Model file for the job. Use its own axes, mm. A direction names the side the tool comes from. Round coordinates to 2 decimals unless told otherwise and drop trailing zeros. Loops run counter-clockwise (first coordinate to the right, second up) from the corner with the lowest first, then second, coordinate; pieces in that order, holes last.
from build123d import *

# Parameters (mm, degrees)
SKETCH1_R           = 2.325
BOSS_EXTRUDE1_DEPTH = 16.05
SKETCH1_3_W         = 4.825
SKETCH1_3_H         = 6.325
SKETCH1_3_R         = 2.325
BOSS_EXTRUDE2_DEPTH = 2.35
SKETCH1_4_R         = 2.325
BOSS_EXTRUDE3_DEPTH = 6.6
SKETCH1_5_R         = 2.325
BOSS_EXTRUDE4_DEPTH = 10.8
SKETCH1_6_R         = 2.325
BOSS_EXTRUDE5_DEPTH = 13.8


with BuildPart() as part:
    # Sketch1 → Boss-Extrude1 (new body)
    # profile 1 of 8: a face of its own
    with BuildSketch(Plane(origin=(0, 0, 0), x_dir=(1, 0, 0), z_dir=(0, 1, 0))):
        with BuildLine():
            Line((-11.4, 0), (-1.25, 0))
            ThreePointArc((-1.25, 0), (-0.929373406, 1.988246715), (0, 3.774917218))
            Line((0, 3.774917218), (0, 6.325))
            Line((0, 6.325), (-11.4, 6.325))
            Line((-11.4, 6.325), (-11.4, 0))
        make_face()
    # profile 2 of 8: a face of its own
    with BuildSketch(Plane(origin=(0, 0, 0), x_dir=(1, 0, 0), z_dir=(0, 1, 0))):
        with BuildLine():
            ThreePointArc((5.075000013, -6.325), (0.602549614, -4.472450396), (-1.25, 0))
            Line((-1.25, 0), (-11.4, 0))
            Line((-11.4, 0), (-11.4, -6.325))
            Line((-11.4, -6.325), (5.075000013, -6.325))
        make_face()
    # profile 3 of 8: a face of its own
    with BuildSketch(Plane(origin=(0, 0, 0), x_dir=(1, 0, 0), z_dir=(0, 1, 0))):
        with BuildLine():
            Line((0, 3.774917218), (0, 0))
            Line((0, 0), (-1.25, 0))
            ThreePointArc((-1.25, 0), (0.602549614, -4.472450396), (5.075000013, -6.325))
            ThreePointArc((5.075000013, -6.325), (9.547450396, -4.472450386), (11.4, 0))
            ThreePointArc((11.4, 0), (9.547450389, 4.472450393), (5.074999993, 6.325))
            ThreePointArc((5.074999993, 6.325), (2.23516958, 5.651635886), (0, 3.774917218))
        make_face()
        with Locations((5.075, 0)):
            Circle(SKETCH1_R, mode=Mode.SUBTRACT)
    # profile 4 of 8: a face of its own
    with BuildSketch(Plane(origin=(0, 0, 0), x_dir=(1, 0, 0), z_dir=(0, 1, 0))):
        with BuildLine():
            Line((-1.25, 0), (0, 0))
            Line((0, 0), (0, 3.774917218))
            ThreePointArc((0, 3.774917218), (-0.929373406, 1.988246715), (-1.25, 0))
        make_face()
    # profile 5 of 8: a face of its own
    with BuildSketch(Plane(origin=(0, 0, 0), x_dir=(1, 0, 0), z_dir=(0, 1, 0))):
        with BuildLine():
            Line((0, 6.325), (0, 3.774917218))
            ThreePointArc((0, 3.774917218), (2.23516958, 5.651635886), (5.074999993, 6.325))
            Line((5.074999993, 6.325), (0, 6.325))
        make_face()
    # profile 6 of 8: a face of its own
    with BuildSketch(Plane(origin=(0, 0, 0), x_dir=(1, 0, 0), z_dir=(0, 1, 0))):
        with BuildLine():
            Line((11.4, 6.325), (5.074999993, 6.325))
            ThreePointArc((5.074999993, 6.325), (9.547450389, 4.472450393), (11.4, 0))
            Line((11.4, 0), (11.4, 6.325))
        make_face()
    # profile 7 of 8: a face of its own
    with BuildSketch(Plane(origin=(0, 0, 0), x_dir=(1, 0, 0), z_dir=(0, 1, 0))):
        with BuildLine():
            ThreePointArc((11.4, 0), (9.547450396, -4.472450386), (5.075000013, -6.325))
            Line((5.075000013, -6.325), (11.4, -6.325))
            Line((11.4, -6.325), (11.4, 0))
        make_face()
    # profile 8 of 8: a face of its own
    with BuildSketch(Plane(origin=(0, 0, 0), x_dir=(1, 0, 0), z_dir=(0, 1, 0))):
        with Locations((5.075, 0)):
            Circle(SKETCH1_R)
    extrude(amount=-BOSS_EXTRUDE1_DEPTH)

    # Sketch1_3 → Boss-Extrude2 (add)
    # profile 1 of 11: a face of its own
    with BuildSketch(Plane(origin=(0, 0, 0), x_dir=(1, 0, 0), z_dir=(0, 1, 0))):
        with Locations((-13.8125, -3.1625)):
            Rectangle(SKETCH1_3_W, SKETCH1_3_H)
    # profile 2 of 11: a face of its own
    with BuildSketch(Plane(origin=(0, 0, 0), x_dir=(1, 0, 0), z_dir=(0, 1, 0))):
        with BuildLine():
            ThreePointArc((5.075000013, -6.325), (0.602549614, -4.472450396), (-1.25, 0))
            Line((-1.25, 0), (-11.4, 0))
            Line((-11.4, 0), (-11.4, -6.325))
            Line((-11.4, -6.325), (5.075000013, -6.325))
        make_face()
    # profile 3 of 11: a face of its own
    with BuildSketch(Plane(origin=(0, 0, 0), x_dir=(1, 0, 0), z_dir=(0, 1, 0))):
        with BuildLine():
            Line((-11.4, 0), (-1.25, 0))
            ThreePointArc((-1.25, 0), (-0.929373406, 1.988246715), (0, 3.774917218))
            Line((0, 3.774917218), (0, 6.325))
            Line((0, 6.325), (-11.4, 6.325))
            Line((-11.4, 6.325), (-11.4, 0))
        make_face()
    # profile 4 of 11: a face of its own
    with BuildSketch(Plane(origin=(0, 0, 0), x_dir=(1, 0, 0), z_dir=(0, 1, 0))):
        with Locations((-13.8125, 3.1625)):
            Rectangle(SKETCH1_3_W, SKETCH1_3_H)
    # profile 5 of 11: a face of its own
    with BuildSketch(Plane(origin=(0, 0, 0), x_dir=(1, 0, 0), z_dir=(0, 1, 0))):
        with BuildLine():
            Line((0, 3.774917218), (0, 0))
            Line((0, 0), (-1.25, 0))
            ThreePointArc((-1.25, 0), (0.602549614, -4.472450396), (5.075000013, -6.325))
            ThreePointArc((5.075000013, -6.325), (9.547450396, -4.472450386), (11.4, 0))
            ThreePointArc((11.4, 0), (9.547450389, 4.472450393), (5.074999993, 6.325))
            ThreePointArc((5.074999993, 6.325), (2.23516958, 5.651635886), (0, 3.774917218))
        make_face()
        with Locations((5.075, 0)):
            Circle(SKETCH1_3_R, mode=Mode.SUBTRACT)
    # profile 6 of 11: a face of its own
    with BuildSketch(Plane(origin=(0, 0, 0), x_dir=(1, 0, 0), z_dir=(0, 1, 0))):
        with Locations((5.075, 0)):
            Circle(SKETCH1_3_R)
    # profile 7 of 11: a face of its own
    with BuildSketch(Plane(origin=(0, 0, 0), x_dir=(1, 0, 0), z_dir=(0, 1, 0))):
        with BuildLine():
            Line((-1.25, 0), (0, 0))
            Line((0, 0), (0, 3.774917218))
            ThreePointArc((0, 3.774917218), (-0.929373406, 1.988246715), (-1.25, 0))
        make_face()
    # profile 8 of 11: a face of its own
    with BuildSketch(Plane(origin=(0, 0, 0), x_dir=(1, 0, 0), z_dir=(0, 1, 0))):
        with BuildLine():
            Line((0, 6.325), (0, 3.774917218))
            ThreePointArc((0, 3.774917218), (2.23516958, 5.651635886), (5.074999993, 6.325))
            Line((5.074999993, 6.325), (0, 6.325))
        make_face()
    # profile 9 of 11: a face of its own
    with BuildSketch(Plane(origin=(0, 0, 0), x_dir=(1, 0, 0), z_dir=(0, 1, 0))):
        with BuildLine():
            Line((11.4, 6.325), (5.074999993, 6.325))
            ThreePointArc((5.074999993, 6.325), (9.547450389, 4.472450393), (11.4, 0))
            Line((11.4, 0), (11.4, 6.325))
        make_face()
    # profile 10 of 11: a face of its own
    with BuildSketch(Plane(origin=(0, 0, 0), x_dir=(1, 0, 0), z_dir=(0, 1, 0))):
        with BuildLine():
            ThreePointArc((11.4, 0), (9.547450396, -4.472450386), (5.075000013, -6.325))
            Line((5.075000013, -6.325), (11.4, -6.325))
            Line((11.4, -6.325), (11.4, 0))
        make_face()
    # profile 11 of 11: a face of its own
    with BuildSketch(Plane(origin=(0, 0, 0), x_dir=(1, 0, 0), z_dir=(0, 1, 0))):
        Polygon((11.4, 0), (11.4, -6.325), (16.225, -6.325), (16.225, 6.325), (11.4, 6.325), align=None)
    extrude(amount=BOSS_EXTRUDE2_DEPTH)

    # Sketch1_4 → Boss-Extrude3 (add)
    # profile 1 of 8: a face of its own
    with BuildSketch(Plane(origin=(0, 0, 0), x_dir=(1, 0, 0), z_dir=(0, 1, 0))):
        with BuildLine():
            Line((-11.4, 0), (-1.25, 0))
            ThreePointArc((-1.25, 0), (-0.929373406, 1.988246715), (0, 3.774917218))
            Line((0, 3.774917218), (0, 6.325))
            Line((0, 6.325), (-11.4, 6.325))
            Line((-11.4, 6.325), (-11.4, 0))
        make_face()
    # profile 2 of 8: a face of its own
    with BuildSketch(Plane(origin=(0, 0, 0), x_dir=(1, 0, 0), z_dir=(0, 1, 0))):
        with BuildLine():
            ThreePointArc((5.075000013, -6.325), (0.602549614, -4.472450396), (-1.25, 0))
            Line((-1.25, 0), (-11.4, 0))
            Line((-11.4, 0), (-11.4, -6.325))
            Line((-11.4, -6.325), (5.075000013, -6.325))
        make_face()
    # profile 3 of 8: a face of its own
    with BuildSketch(Plane(origin=(0, 0, 0), x_dir=(1, 0, 0), z_dir=(0, 1, 0))):
        with BuildLine():
            Line((0, 3.774917218), (0, 0))
            Line((0, 0), (-1.25, 0))
            ThreePointArc((-1.25, 0), (0.602549614, -4.472450396), (5.075000013, -6.325))
            ThreePointArc((5.075000013, -6.325), (9.547450396, -4.472450386), (11.4, 0))
            ThreePointArc((11.4, 0), (9.547450389, 4.472450393), (5.074999993, 6.325))
            ThreePointArc((5.074999993, 6.325), (2.23516958, 5.651635886), (0, 3.774917218))
        make_face()
        with Locations((5.075, 0)):
            Circle(SKETCH1_4_R, mode=Mode.SUBTRACT)
    # profile 4 of 8: a face of its own
    with BuildSketch(Plane(origin=(0, 0, 0), x_dir=(1, 0, 0), z_dir=(0, 1, 0))):
        with BuildLine():
            Line((0, 6.325), (0, 3.774917218))
            ThreePointArc((0, 3.774917218), (2.23516958, 5.651635886), (5.074999993, 6.325))
            Line((5.074999993, 6.325), (0, 6.325))
        make_face()
    # profile 5 of 8: a face of its own
    with BuildSketch(Plane(origin=(0, 0, 0), x_dir=(1, 0, 0), z_dir=(0, 1, 0))):
        with BuildLine():
            Line((11.4, 6.325), (5.074999993, 6.325))
            ThreePointArc((5.074999993, 6.325), (9.547450389, 4.472450393), (11.4, 0))
            Line((11.4, 0), (11.4, 6.325))
        make_face()
    # profile 6 of 8: a face of its own
    with BuildSketch(Plane(origin=(0, 0, 0), x_dir=(1, 0, 0), z_dir=(0, 1, 0))):
        with BuildLine():
            ThreePointArc((11.4, 0), (9.547450396, -4.472450386), (5.075000013, -6.325))
            Line((5.075000013, -6.325), (11.4, -6.325))
            Line((11.4, -6.325), (11.4, 0))
        make_face()
    # profile 7 of 8: a face of its own
    with BuildSketch(Plane(origin=(0, 0, 0), x_dir=(1, 0, 0), z_dir=(0, 1, 0))):
        with BuildLine():
            Line((-1.25, 0), (0, 0))
            Line((0, 0), (0, 3.774917218))
            ThreePointArc((0, 3.774917218), (-0.929373406, 1.988246715), (-1.25, 0))
        make_face()
    # profile 8 of 8: a face of its own
    with BuildSketch(Plane(origin=(0, 0, 0), x_dir=(1, 0, 0), z_dir=(0, 1, 0))):
        with Locations((5.075, 0)):
            Circle(SKETCH1_4_R)
    extrude(amount=BOSS_EXTRUDE3_DEPTH)

    # Sketch1_5 → Boss-Extrude4 (add)
    # profile 1 of 3: a face of its own
    with BuildSketch(Plane(origin=(0, 0, 0), x_dir=(1, 0, 0), z_dir=(0, 1, 0))):
        with BuildLine():
            Line((0, 3.774917218), (0, 0))
            Line((0, 0), (-1.25, 0))
            ThreePointArc((-1.25, 0), (0.602549614, -4.472450396), (5.075000013, -6.325))
            ThreePointArc((5.075000013, -6.325), (9.547450396, -4.472450386), (11.4, 0))
            ThreePointArc((11.4, 0), (9.547450389, 4.472450393), (5.074999993, 6.325))
            ThreePointArc((5.074999993, 6.325), (2.23516958, 5.651635886), (0, 3.774917218))
        make_face()
        with Locations((5.075, 0)):
            Circle(SKETCH1_5_R, mode=Mode.SUBTRACT)
    # profile 2 of 3: a face of its own
    with BuildSketch(Plane(origin=(0, 0, 0), x_dir=(1, 0, 0), z_dir=(0, 1, 0))):
        with Locations((5.075, 0)):
            Circle(SKETCH1_5_R)
    # profile 3 of 3: a face of its own
    with BuildSketch(Plane(origin=(0, 0, 0), x_dir=(1, 0, 0), z_dir=(0, 1, 0))):
        with BuildLine():
            Line((-1.25, 0), (0, 0))
            Line((0, 0), (0, 3.774917218))
            ThreePointArc((0, 3.774917218), (-0.929373406, 1.988246715), (-1.25, 0))
        make_face()
    extrude(amount=BOSS_EXTRUDE4_DEPTH)

    # Sketch1_6 → Boss-Extrude5 (add)
    with BuildSketch(Plane(origin=(0, 0, 0), x_dir=(1, 0, 0), z_dir=(0, 1, 0))):
        with Locations(Location((5.075, 0, 0), (0, 0, 90))):
            Circle(SKETCH1_6_R)
    extrude(amount=BOSS_EXTRUDE5_DEPTH)


solid = part.part
Q1. Slice it at A-A on z = -1. Give the cut face in (x, y) (3 decimals), plus the area to 3 significant figures.
Q2. Slice it at B-B on x = 6.5. Give the cut face in (y, z) (3 decimals), plus the area to 3 significant figures.
Q3. Slice it at C-C on y = -3. Give the cut face in (x, z) (3 decimals).
Q4. Tool access for faces 1 (the face through (10, 6.6, 5)), 2 (the face through (14, 0, 0)), 3 (the face through (5, 10.8, 3)), 4 (the face through (-14, 2.35, 0)): list every direction of +Z, -Z, +X, -X, +Y, -Y with a clear straight run to the whole face (end or side of a thin tool).
Q5. Probe line 1 (X direction, y = -9.75, z = -4); line 2 (Y direction, x = 9, z = -3.75); line 3 (Y direction, x = 13, z = 5.5). List the from-to ranges inside material, lowest first.
Q6. Flat gauge pins, fed straight in: P1, Ø1.3, axis at y = 4, z = 2.5, coming from the +X side; P2, Ø4, axis at x = -1.5, y = 9, coming from the -Z side; P3, Ø3, axis at x = 8, z = -4, coming from the +Y side. Where does each tip first touch, or does it go through?
Q7. Slice it at D-D on z = 1.5. Give the cut face in (x, y) (3 decimals).
Reply:
1. outline: (-16.225, 0) - (-11.4, 0) - (-11.4, -16.05) - (11.4, -16.05) - (11.4, 0) - (16.225, 0) - (16.225, 2.35) - (11.4, 2.35) - (11.4, 6.6) - (11.32, 6.6) - (11.32, 10.8) - (7.174, 10.8) - (7.174, 13.8) - (2.976, 13.8) - (2.976, 10.8) - (-1.17, 10.8) - (-1.17, 6.6) - (-11.4, 6.6) - (-11.4, 2.35) - (-16.225, 2.35) - close
1. area: 604 mm2
2. outline: (-16.05, -6.325) - (6.6, -6.325) - (6.6, -6.162) - (10.8, -6.162) - (10.8, -1.837) - (13.8, -1.837) - (13.8, 1.837) - (10.8, 1.837) - (10.8, 6.162) - (6.6, 6.162) - (6.6, 6.325) - (-16.05, 6.325) - close
2. area: 349 mm2
3. outline: (-11.4, -6.325) - (11.4, -6.325) - (11.4, 6.325) - (-11.4, 6.325) - close
4. face 1: +Z, +X, +Y
4. face 2: +Z, -Z, +X, -Y
4. face 3: +Y
4. face 4: +Z, -Z, -X, +Y
5. line 1: x = -11.4 to 11.4
5. line 2: y = -16.05 to 10.8
5. line 3: y = 0 to 2.35
6. P1: stops at x = 11.4
6. P2: stops at z = -4.37
6. P3: stops at y = 10.8
7. outline: (-16.225, 0) - (-11.4, 0) - (-11.4, -16.05) - (11.4, -16.05) - (11.4, 0) - (16.225, 0) - (16.225, 2.35) - (11.4, 2.35) - (11.4, 6.6) - (11.22, 6.6) - (11.22, 10.8) - (6.851, 10.8) - (6.851, 13.8) - (3.299, 13.8) - (3.299, 10.8) - (-1.07, 10.8) - (-1.07, 6.6) - (-11.4, 6.6) - (-11.4, 2.35) - (-16.225, 2.35) - close
